Build history of the part. All positions in model axes, mm. Face numbers are marked on the shaded views. A direction names the side the tool comes from. Give positions to 0.01 mm unless a question says otherwise; leave off trailing zeros. Write each loop counter-clockwise with the first axis right and the second up, starting at its lowest first coordinate (ties: lowest second). Pieces come first, ordered by that corner, then holes.
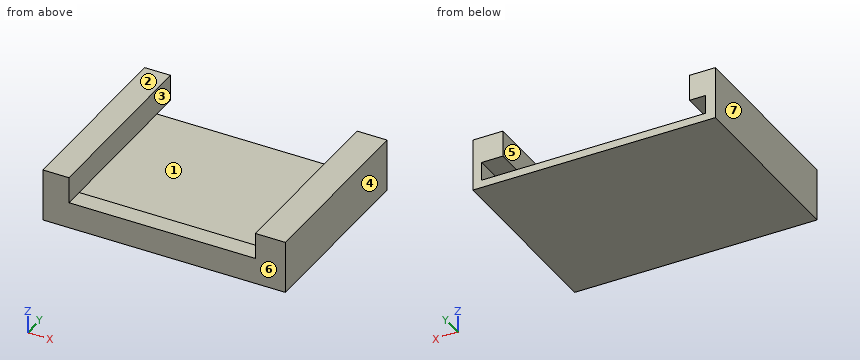
from build123d import *

# Parameters (mm, degrees)
SKETCH1_W           = 13
SKETCH1_H           = 28
BOSS_EXTRUDE1_DEPTH = 10
CUT_EXTRUDE1_DEPTH  = 9
CUT_EXTRUDE3_DEPTH  = 19.391574158


with BuildPart() as part:
    # Sketch1 → Boss-Extrude1 (new body)
    with BuildSketch(Plane(origin=(0, 0, 0), x_dir=(1, 0, 0), z_dir=(0, 1, 0))):
        Rectangle(SKETCH1_W, SKETCH1_H)
    extrude(amount=BOSS_EXTRUDE1_DEPTH)

    # Sketch2 → Cut-Extrude1 (cut)
    with BuildSketch(Plane(origin=(0, 10, 0), x_dir=(1, 0, 0), z_dir=(0, 1, 0))):
        Polygon((0, 13.590584793), (-5.963515209, 13.590584793), (-5.963515209, 12.590584793), (6.036484791, 12.590584793), (6.036484791, 13.590584793), align=None)
    extrude(amount=-CUT_EXTRUDE1_DEPTH, mode=Mode.SUBTRACT)

    # Sketch3 → Cut-Extrude3 (cut, through all)
    with BuildSketch(Plane(origin=(0, 10, 0), x_dir=(1, 0, 0), z_dir=(0, 1, 0))):
        Polygon((-5.107870795, 12.590584793), (-5.107870795, 11.182588561), (-6.5, 11.182588561), (-6.5, -14), (6.5, -14), (6.5, 11.182588561), (4.888962046, 11.182588561), (4.888962046, 12.590584793), align=None)
    extrude(amount=-CUT_EXTRUDE3_DEPTH, mode=Mode.SUBTRACT)


solid = part.part
1. Saw through at B-B on y = 3.25. Give the cut face in (x, z), plus the area to 3 significant figures.
2. 3-axis set-ups, long thin cutter, end or side, ignore diameter. For the marked faces 1, 2 and 3: which of +Z, -Z, +X, -X, +Y, -Y reach the whole face in a straight line?
3. Saw through at A-A on z = -12.2. Give the cut face in (x, y).
4. Drill centre lines: line 1 along X through (y, z) = (9, -12.35); line 2 along X through (y, z) = (6.5, -13.25); line 3 along Z through (x, y) = (5.25, 5.75). Where is each one in solid material? Low to high.
5. Drop flat-ended pins along their axis: pin 1 (1.5 mm diameter, centred on x = 0.5, y = 9, fed in from +Z); pin 2 (0.5 mm diameter, centred on x = 2, z = -13, fed in from +Y). Give the stop position or say it passes through.
6. Saw through at C-C on z = -13. Give the cut face in (x, y).
7. Saw through at D-D on x = 4.25. Give the cut face in (y, z).
8. Mould opens along X. For the marked faces 4, 5, 6 and 7 say: pulls with the +X half, pulls with the -X half, needs draft (parallel to the pull), parting line crosses it, or undercut.
Outcome:
1. outline: (-6.5, -14) - (6.5, -14) - (6.5, -11.18) - (4.89, -11.18) - (4.89, -12.59) - (6.04, -12.59) - (6.04, -13.59) - (-5.96, -13.59) - (-5.96, -12.59) - (-5.11, -12.59) - (-5.11, -11.18) - (-6.5, -11.18) - close
1. area: 10.6 mm2
2. face 1: +Y
2. face 2: +Z, +X, -X, +Y, -Y
2. face 3: +Z, +Y, -Y
3. outline: (-6.5, 0) - (-5.11, 0) - (-5.11, 10) - (-6.5, 10) - close; (4.89, 0) - (6.5, 0) - (6.5, 10) - (4.89, 10) - close
4. line 1: x = -6.5 to -5.11, 4.89 to 6.5
4. line 2: x = -6.5 to -5.96, 6.04 to 6.5
4. line 3: z = -14 to -13.59, -12.59 to -11.18
5. pin 1: stops at z = -13.59
5. pin 2: stops at y = 1
6. outline: (-6.5, 0) - (6.5, 0) - (6.5, 10) - (6.04, 10) - (6.04, 1) - (-5.96, 1) - (-5.96, 10) - (-6.5, 10) - close
7. outline: (0, -14) - (10, -14) - (10, -13.59) - (1, -13.59) - (1, -12.59) - (0, -12.59) - close
8. face 4: pulls with the +X half
8. face 5: undercut
8. face 6: needs draft
8. face 7: pulls with the -X half
